```python
from build123d import *

# Parameters (mm, degrees)
BOSS_EXTRUDE1_DEPTH = 10
CUT_EXTRUDE3_DEPTH  = 68.292273107
CHAMFER2_SIZE       = 1.5
SKETCH2_R           = 3.5
CUT_EXTRUDE1_DEPTH  = 1.5
SKETCH3_R           = 1.5
CUT_EXTRUDE2_DEPTH  = 68.007462417
CHAMFER1_SIZE       = 1.5


with BuildPart() as part:
    # Sketch1 → Boss-Extrude1 (new, symmetric)
    with BuildSketch(Plane.XY):
        Polygon((-58, 0), (58, 0), (58, -10), (61, -7), (61, 3.5), (-61, 3.5), (-61, -7), (-58, -10), align=None)
    extrude(amount=BOSS_EXTRUDE1_DEPTH, both=True)

    # Sketch4 → section 0 of loft1
    with BuildSketch(Plane.XY.offset(-25), mode=Mode.PRIVATE) as loft1_s0:
        with BuildLine():
            Line((58, -2.928932188), (61, 0.071067812))
            Line((61, 0.071067812), (61, 3.5))
            Line((61, 3.5), (-61, 3.5))
            Line((-61, 3.5), (-61, 0.071067812))
            Line((-61, 0.071067812), (-58, -2.928932188))
            Line((-58, -2.928932188), (-58, 0))
            Line((-58, 0), (58, 0))
            Line((58, 0), (58, -2.928932188))
        make_face()
    # loft up to a face of the part (loft1)
    loft([loft1_s0.sketch, part.faces().sort_by_distance((0, 1.105125523, -10))[0]])

    # Sketch5 → section 1 of loft2
    with BuildSketch(Plane.XY.offset(25), mode=Mode.PRIVATE) as loft2_s1:
        with BuildLine():
            Line((-58, 0), (58, 0))
            Line((58, 0), (58, -2.928932188))
            Line((58, -2.928932188), (61, 0.071067812))
            Line((61, 0.071067812), (61, 3.5))
            Line((61, 3.5), (-61, 3.5))
            Line((-61, 3.5), (-61, 0.071067812))
            Line((-61, 0.071067812), (-58, -2.928932188))
            Line((-58, -2.928932188), (-58, 0))
        make_face()
    # loft from a face of the part (loft2)
    loft([part.faces().sort_by_distance((0, 1.105125523, 10))[0], loft2_s1.sketch])

    # Sketch6 → Cut-Extrude3 (cut, through all)
    with BuildSketch(Plane(origin=(0, 3.5, 0), x_dir=(1, 0, 0), z_dir=(0, 1, 0))):
        Polygon((43.107671767, 5), (-43.107671767, 5), (-53.5, 15.392328233), (-52.687543149, 20), (52.687543149, 20), (53.5, 15.392328233), align=None)
        Polygon((43.107671767, -5), (-43.107671767, -5), (-53.5, -15.392328233), (-52.687543149, -20), (52.687543149, -20), (53.5, -15.392328233), align=None)
    extrude(amount=-CUT_EXTRUDE3_DEPTH, mode=Mode.SUBTRACT)

    # Chamfer2
    chamfer2_edges = [part.edges().sort_by_distance(p)[0] for p in [
        (48.303835883, 3.5, -10.196164117),
        (53.093771575, 3.5, -17.696164117),
        (0, 3.5, -20),
        (-53.093771575, 3.5, -17.696164117),
        (-48.303835883, 3.5, -10.196164117),
        (0, 3.5, -5),
        (-53.093771575, 3.5, 17.696164117),
        (0, 3.5, 20),
        (53.093771575, 3.5, 17.696164117),
        (48.303835883, 3.5, 10.196164117),
        (0, 3.5, 5),
        (-48.303835883, 3.5, 10.196164117),
        (-61, 3.5, 0),
        (61, 3.5, 0),
        (0, 3.5, -25),
        (0, 3.5, 25),
    ]]
    chamfer(chamfer2_edges, length=CHAMFER2_SIZE)

    # Sketch2 → Cut-Extrude1 (cut)
    with BuildSketch(Plane(origin=(0, 3.5, 0), x_dir=(1, 0, 0), z_dir=(0, 1, 0))):
        with Locations(Location((49, 0, 0), (0, 0, 270))):
            Circle(SKETCH2_R)
        with Locations(Location((-49, 0, 0), (0, 0, 270))):
            Circle(SKETCH2_R)
    extrude(amount=-CUT_EXTRUDE1_DEPTH, mode=Mode.SUBTRACT)

    # Sketch3 → Cut-Extrude2 (cut, through all)
    with BuildSketch(Plane(origin=(0, 2, 0), x_dir=(1, 0, 0), z_dir=(0, 1, 0))):
        with Locations(Location((49, 0, 0), (0, 0, 180))):
            Circle(SKETCH3_R)
        with Locations(Location((-49, 0, 0), (0, 0, 180))):
            Circle(SKETCH3_R)
    extrude(amount=-CUT_EXTRUDE2_DEPTH, mode=Mode.SUBTRACT)

    # Chamfer1
    chamfer1_edges = [part.edges().sort_by_distance(p)[0] for p in [
        (50.5, 2, 0),
        (-47.5, 2, 0),
    ]]
    chamfer(chamfer1_edges, length=CHAMFER1_SIZE)


solid = part.part
```
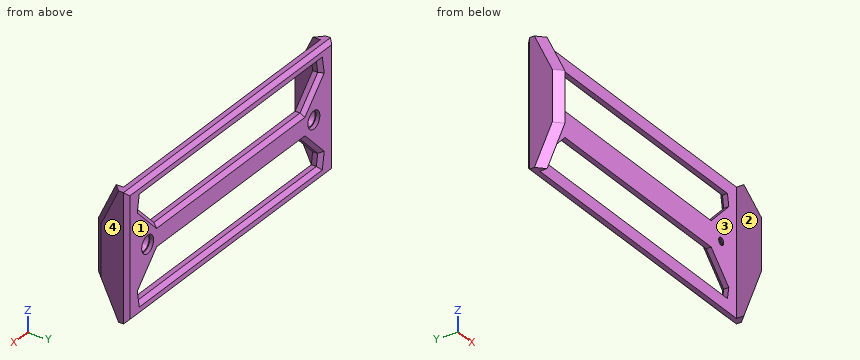
Build history of the part. All positions in model axes, mm. Face numbers are marked on the shaded views. Round coordinates to 2 decimals unless told otherwise and drop trailing zeros. Order: outer loops, then holes, each group sorted by start corner. A loop starts at its lowest first (then second) coordinate and runs counter-clockwise, first axis right, second up. Notation, with made-up numbers: (76.5, -38.5) - (125.5, -38.5) arc R23 ccw to (125.5, -1.5) - close; hole circle Ø6 at (-20.5, 22). An arc over 180 degrees is marked (long way). Use a Markdown table: item, result.
1) Saw through at C-C on x = 49. Write the cut outline in (y, z).
Recorded:
| item | result |
|---|---|
| outline | (0, -25) - (2, -25) - (3.5, -23.5) - (3.5, -21.5) - (2, -20) - (0, -20) - close; (0, -10.89) - (2, -10.89) - (3.5, -8.77) - (3.5, -3.5) - (2, -3.5) - (2, -3) - (0.5, -1.5) - (0, -1.5) - close; (0, 1.5) - (0.5, 1.5) - (2, 3) - (2, 3.5) - (3.5, 3.5) - (3.5, 8.77) - (2, 10.89) - (0, 10.89) - close; (0, 20) - (2, 20) - (3.5, 21.5) - (3.5, 23.5) - (2, 25) - (0, 25) - close |
2) Saw through at B-B on z = 0. Give the number of separate pieces and of enclosed holes in the cut face, and give its area (3 significant figures).
Recorded:
| item | result |
|---|---|
| separate pieces | 3 |
| enclosed holes | 0 |
| area | 438 mm² |
3) Saw through at D-D on z = -6.5. Write the cut outline in (x, y), and give its area (3 significant figures).
Recorded:
| item | result |
|---|---|
| outline | (-61, -7) - (-58, -10) - (-58, 0) - (-44.61, 0) - (-44.61, 2) - (-46.73, 3.5) - (-59.5, 3.5) - (-61, 2) - close; (44.61, 0) - (58, 0) - (58, -10) - (61, -7) - (61, 2) - (59.5, 3.5) - (46.73, 3.5) - (44.61, 2) - close |
| area | 160 mm² |
4) Saw through at A-A on x = -33. Write the cut outline in (y, z).
Recorded:
| item | result |
|---|---|
| outline | (0, -25) - (2, -25) - (3.5, -23.5) - (3.5, -21.5) - (2, -20) - (0, -20) - close; (0, -5) - (2, -5) - (3.5, -3.5) - (3.5, 3.5) - (2, 5) - (0, 5) - close; (0, 20) - (2, 20) - (3.5, 21.5) - (3.5, 23.5) - (2, 25) - (0, 25) - close |
5) Flat gauge pins, fed straight in: pin 1 Ø9 at (x, z) = (49, 0) entering from -Y; pin 2 Ø3.5 at (x, z) = (-49, 0) entering from +Y. Where does each tip first touch, or does it go through?
Recorded:
| item | result |
|---|---|
| pin 1 | stops at y = 0 |
| pin 2 | stops at y = 0.75 |
6) Wall check: L1, parallel to Z at x = 22.5, y = 1.5; L2, parallel to X at y = -2.25, z = -18; L3, parallel to X at y = 0.25, z = 15.5. Give the ranges that are in metal, low to high.
Recorded:
| item | result |
|---|---|
| L1 | z = -25 to -20, -5 to 5, 20 to 25 |
| L2 | x = -61 to -58, 58 to 61 |
| L3 | x = -61 to -53.48, 53.48 to 61 |
7) Pull direction X, two halves, no side cores. Call the marked faces 1, 2, 3 and 4: pulls with the +X half, pulls with the -X half, needs draft (parallel to the pull), parting line crosses it, or undercut.
Recorded:
| item | result |
|---|---|
| face 1 | needs draft |
| face 2 | undercut |
| face 3 | undercut |
| face 4 | pulls with the +X half |
